Geometry: see drawing. Coordinates: mm, zero at the bounding-box minimum. Give positions to 0.01 mm unless a question says otherwise; leave off trailing zeros. Loops run counter-clockwise (first coordinate to the right, second up) from the corner with the lowest first, then second, coordinate; pieces in that order, holes last. Notation, with made-up numbers: M -21,-32.75 L -8,-32.75 A27 ccw -8,-1.75 Z; hole C 50.25,53 d7. An arc over 180 degrees is marked long. Use CSV: the item, a comma, the result in double quotes. Start each with the question number.
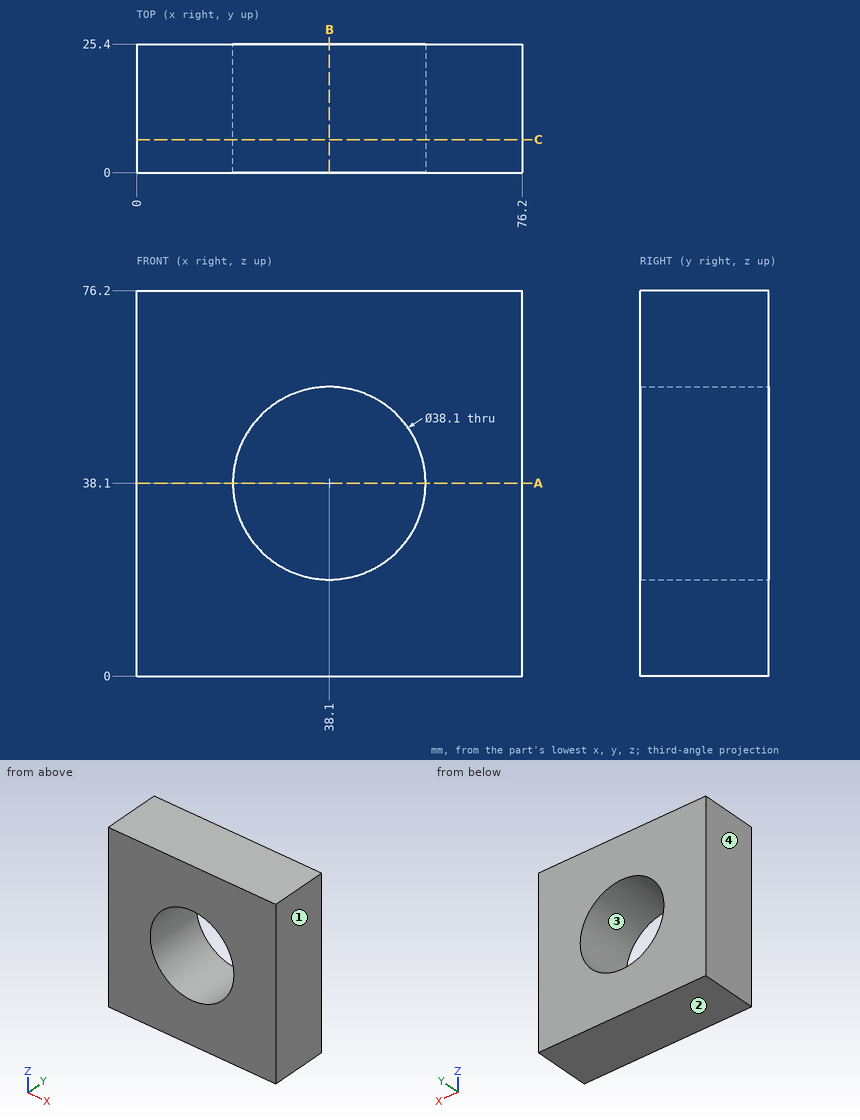
Item 1: Material intervals for line 1 (Z direction, x = 38.1, y = 15); line 2 (X direction, y = 5.25, z = 33.5); line 3 (Z direction, x = 29, y = 13.5), sorted ascending.
Item 2: Section C-C (y = 6.5). Output: boundary loops of the cut face in (x, z).
Item 3: Section A-A (z = 38.1). Output: boundary loops of the cut face in (x, y), then the cut area to 3 significant figures.
Item 4: Mould query, pull axis X, two halves, no side actions, for the marked faces 1, 2, 3 and 4. Classes: +X half, -X half, draft (parallel to the pull), parting line (faces both ways), or undercut.
Item 5: Section B-B (x = 38.1). Output: boundary loops of the cut face in (y, z).
Recorded:
1,line 1,"0 to 19.05, 57.15 to 76.2"
1,line 2,"0 to 19.61, 56.59 to 76.2"
1,line 3,"0 to 21.36, 54.84 to 76.2"
2,outline,"M 0,0 L 76.2,0 L 76.2,76.2 L 0,76.2 Z; hole C 38.1,38.1 d38.1"
3,outline,"M 0,0 L 19.05,0 L 19.05,25.4 L 0,25.4 Z; M 57.15,0 L 76.2,0 L 76.2,25.4 L 57.15,25.4 Z"
3,area,"968 mm²"
4,face 1,"+X half"
4,face 2,"draft"
4,face 3,"undercut"
4,face 4,"-X half"
5,outline,"M 0,0 L 25.4,0 L 25.4,19.05 L 0,19.05 Z; M 0,57.15 L 25.4,57.15 L 25.4,76.2 L 0,76.2 Z"
